Input: part model. Units: mm. Frame: model coordinates. Face numbers are marked on the shaded views. Give positions to 0.01 mm unless a question says otherwise; leave off trailing zeros. Loops run counter-clockwise (first coordinate to the right, second up) from the corner with the lowest first, then second, coordinate; pieces in that order, holes last. Notation, with made-up numbers: M 63.5,12 L 71.5,12 A37 cw 71.5,49 Z; hole C -38.75,16.25 d7. An arc over 180 degrees is marked long. Answer as a JSON object with one key per item and string values. Group by question number.
1) Ray query, L1, parallel to Y at x = 0, z = 1.75; L2, parallel to Y at x = 0, z = 3.05; L3, parallel to X at y = -1, z = 3.75. Return the intervals inside material, ascending.
2) Section query A-A on y = 2. Return loops of the section in (x, z).
3) Section query B-B on x = 0. Return loops of the section in (y, z), plus the area to 3 significant figures.
4) Draft query along X for the marked faces 1, 2 and 3. Return one class per face: +X half, -X half, draft (parallel to the pull), parting line (faces both ways), or undercut.
from build123d import *

# Parameters (mm, degrees)
SKETCH_R  = 2.5
PAD_DEPTH = 4.2
FILLET_R  = 2.5


with BuildPart() as part:
    # Sketch → Pad (new body)
    with BuildSketch(Plane.XY):
        with BuildLine():
            Line((-5.9, 2.9), (-5.9, -2.9))
            ThreePointArc((-5.9, -2.9), (-5.02132, -5.02132), (-2.9, -5.9))
            Line((-2.9, -5.9), (2.9, -5.9))
            ThreePointArc((2.9, -5.9), (5.02132, -5.02132), (5.9, -2.9))
            Line((5.9, -2.9), (5.9, 2.9))
            ThreePointArc((5.9, 2.9), (5.02132, 5.02132), (2.9, 5.9))
            Line((2.9, 5.9), (-2.9, 5.9))
            ThreePointArc((-2.9, 5.9), (-5.02132, 5.02132), (-5.9, 2.9))
        make_face()
        Circle(SKETCH_R, mode=Mode.SUBTRACT)
    extrude(amount=PAD_DEPTH)

    # Fillet
    fillet_edges = [part.edges().sort_by_distance(p)[0] for p in [
        (5.9, 0, 4.2),
    ]]
    fillet(fillet_edges, radius=FILLET_R)


solid = part.part
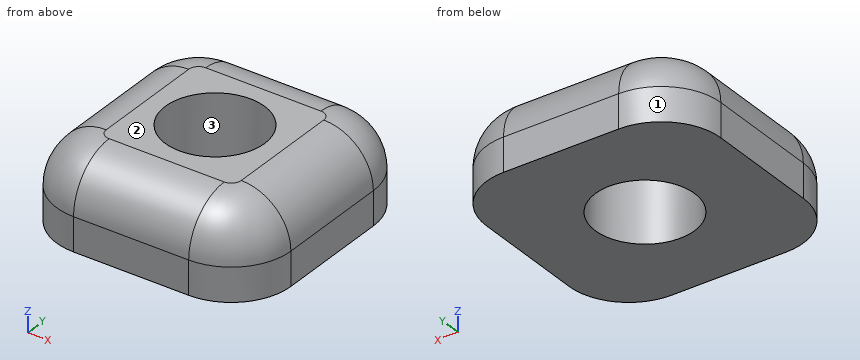
Output:
{
 "1": {"L1": "y = -5.9 to -2.5, 2.5 to 5.9", "L2": "y = -5.5 to -2.5, 2.5 to 5.5", "L3": "x = -4.83 to -2.29, 2.29 to 4.83"},
 "2": {"outline": "M -5.9,0 L -1.5,0 L -1.5,4.2 L -3.4,4.2 A2.5 ccw -5.9,1.7 Z; M 1.5,0 L 5.9,0 L 5.9,1.7 A2.5 ccw 3.4,4.2 L 1.5,4.2 Z"},
 "3": {"outline": "M -5.9,0 L -2.5,0 L -2.5,4.2 L -3.4,4.2 A2.5 ccw -5.9,1.7 Z; M 2.5,0 L 5.9,0 L 5.9,1.7 A2.5 ccw 3.4,4.2 L 2.5,4.2 Z", "area": "25.9 mm^2"},
 "4": {"face 1": "-X half", "face 2": "draft", "face 3": "undercut"}
}
